Part model, mm, in its own coordinate system. A direction names the side the tool comes from. Round coordinates to 2 decimals unless told otherwise and drop trailing zeros. Loops run counter-clockwise (first coordinate to the right, second up) from the corner with the lowest first, then second, coordinate; pieces in that order, holes last. Notation, with made-up numbers: (-35, -9) - (22, -9) arc R30 cw to (22, 24) - close; hole circle Ø3 at (75, -5). An arc over 180 degrees is marked (long way). Put each result on its own line as item: value.
from build123d import *


with BuildPart() as part:
    # Эскиз1 → Повернуть1 (revolve)
    with BuildSketch(Plane(origin=(0, 0, 0), x_dir=(0, 0, -1), z_dir=(1, 0, 0))):
        with BuildLine():
            Line((-37.5, 0), (-37.5, 4))
            Line((-37.5, 4), (-7.5, 4))
            Line((-7.5, 4), (-7.5, 10.5))
            Line((-7.5, 10.5), (-1.5, 10.5))
            Line((-1.5, 10.5), (-1.5, 5))
            Line((-1.5, 5), (0, 5))
            Line((0, 5), (0, 10.5))
            Line((0, 10.5), (6, 10.5))
            Line((6, 10.5), (6, 5))
            Line((6, 5), (10, 5))
            Line((10, 5), (10, 9.516531243))
            ThreePointArc((10, 9.516531243), (10.281302062, 10.211853667), (10.966946547, 10.515984828))
            ThreePointArc((10.966946547, 10.515984828), (21.86672187, 13.014935813), (31.032522672, 19.421023056))
            ThreePointArc((31.032522672, 19.421023056), (31.622642119, 19.717638439), (32.268965333, 19.581668037))
            Line((32.268965333, 19.581668037), (34.156309404, 18.440297549))
            ThreePointArc((34.156309404, 18.440297549), (34.606360099, 17.837352598), (34.508702483, 17.091328984))
            ThreePointArc((34.508702483, 17.091328984), (31.146131827, 8.838013416), (30, 0))
            Line((30, 0), (-37.5, 0))
        make_face()
    revolve(axis=Axis((0, 0, 37.5), (0, 0, -1)))


solid = part.part
1. Probe line 1 along Z through (x, y) = (-9.5, 3.5); line 2 along Z through (x, y) = (-2, -6); line 3 along Z through (x, y) = (-15.5, -6.5). List the from-to ranges inside material, lowest first. Write a range as [from, to].
A:
line 1: z = [-31.51, -10.21], [-6, 0], [1.5, 7.5]
line 2: z = [-30.58, -10], [-6, 0], [1.5, 7.5]
line 3: z = [-34.35, -28.15]
2. Band-saw the part on C-C (z = 13). List the corners of the cut face in (x, y), plus the area to 3 significant figures.
A:
outline: circle Ø8 at (0, 0)
area: 50.3 mm²
3. Two-plate mould, pull along Z, no slides. Class faces 4 (the flat face through (0, -5, 7.5)), 5 (the flat face through (-2, 5, 1.5)), 6 (the cylindrical face through (3.2, 10, -3)): pulls with the +Z half, pulls with the -Z half, needs draft (parallel to the pull), parting line crosses it, or undercut.
A:
face 4: pulls with the +Z half
face 5: undercut
face 6: needs draft
4. Tool access for faces 1 (the cylindrical face through (-3.905, -0.867, 22.29)), 2 (the flat face through (0, 0, 37.5)), 3 (the flat face through (-4, -4, -10)): list every direction of +Z, -Z, +X, -X, +Y, -Y with a clear straight run to the whole face (end or side of a thin tool).
A:
face 1: +Z
face 2: +Z, +X, -X, +Y, -Y
face 3: none
5. Pin check, flat tips, straight feed: P1, Ø17, axis at x = 5, y = -4, coming from the +Z side; P2, Ø6, axis at x = 6.5, z = -27, coming from the +Y side; P3, Ø2, axis at y = -10.5, z = -26.5, coming from the +X side; P4, Ø23, axis at x = -4.5, y = -1.5, coming from the -Z side. Stop position of each tip, or through.
A:
P1: stops at z = 37.5
P2: stops at y = 17.4
P3: stops at x = 12.78
P4: stops at z = -34.04
6. Band-saw the part on D-D (z = -7). List the corners of the cut face in (x, y).
A:
outline: circle Ø10 at (0, 0)
